Answer from the drawing. Dimensions are ordinates in mm from the lowest x, y and z of the part. Give positions to 0.01 mm unless a question says otherwise; leave off trailing zeros. Order: outer loops, then holes, each group sorted by start corner. A loop starts at its lowest first (then second) coordinate and runs counter-clockwise, first axis right, second up. Notation, with made-up numbers: M 2,40.5 L 60,40.5 A15 ccw 60,53.5 Z; hole C 82,-7.5 d5. An arc over 180 degrees is marked long. One line per item, written item: value.
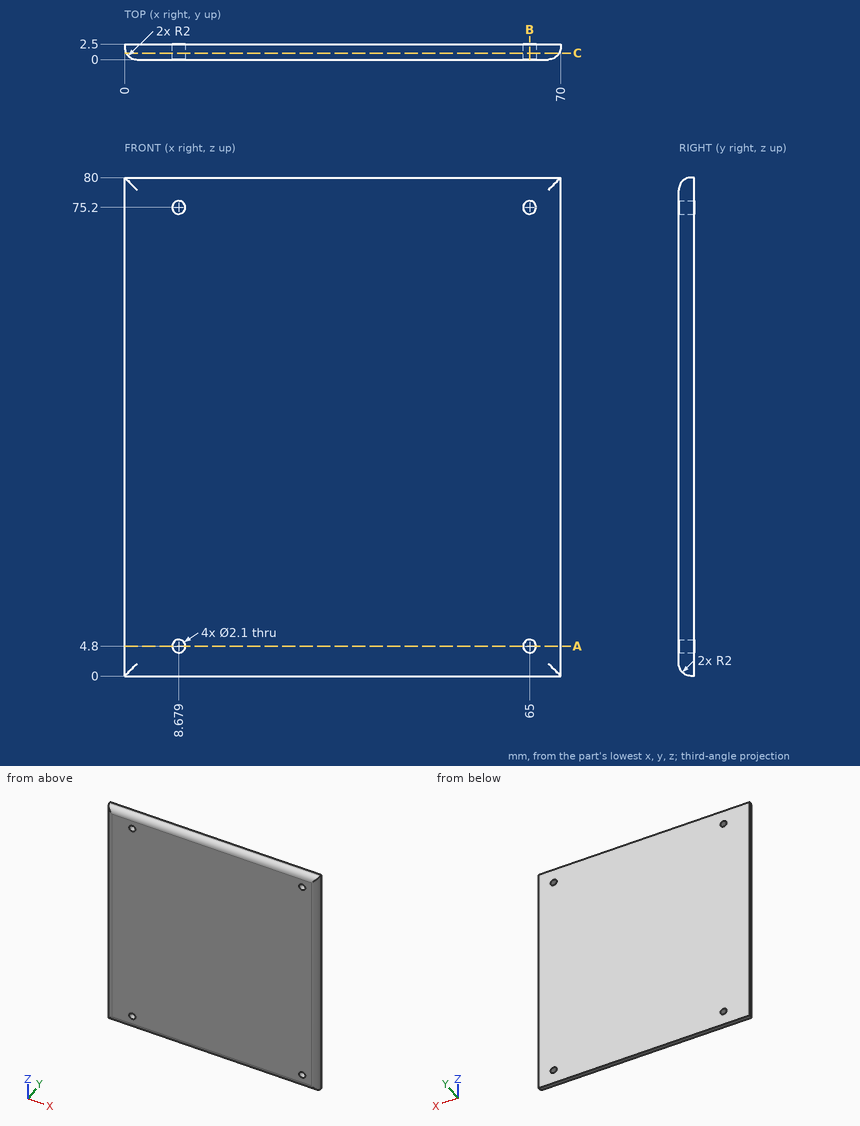
(1) Section B-B, the plane x = 65 is taken. Give the vertices of the cut face in (y, z), then the cut area to 3 significant figures.
Findings:
outline: M 0,2 A2 ccw 2,0 L 2.5,0 L 2.5,3.75 L 0,3.75 Z; M 0,5.85 L 2.5,5.85 L 2.5,74.15 L 0,74.15 Z; M 0,76.25 L 2.5,76.25 L 2.5,80 L 2,80 A2 ccw 0,78 Z
area: 188 mm^2
(2) Given P1, Ø3.5, axis at x = 65, z = 4.8, coming from the -Y side; P2, Ø1.5, axis at x = 18.5, y = 1, coming from the -Z side; P3, Ø1.5, axis at y = 0.5, z = 33, coming from the +X side, each flat-ended and moving along its own axis, determine where each tip first touches the part or whether it passes through.
Findings:
P1: stops at y = 0
P2: stops at z = 0.02
P3: stops at x = 69.85
(3) Section A-A, the plane z = 4.8 is taken. Give the vertices of the cut face in (x, y), then the cut area to 3 significant figures.
Findings:
outline: M 0,2 A2 ccw 2,0 L 7.63,0 L 7.63,2.5 L 0,2.5 Z; M 9.73,0 L 63.95,0 L 63.95,2.5 L 9.73,2.5 Z; M 66.05,0 L 68,0 A2 ccw 70,2 L 70,2.5 L 66.05,2.5 Z
area: 163 mm^2
(4) Find the intervals of material crossed by probe 1 along Z at (x, y) = (65, 1.8); probe 2 along X at (y, z) = (1.55, 75.2); probe 3 along Z at (x, y) = (65, 0.6), in increasing order. Write a range as from..to.
Findings:
probe 1: z = 0.01..3.75, 5.85..74.15, 76.25..79.99
probe 2: x = 0.05..7.63, 9.73..63.95, 66.05..69.95
probe 3: z = 0.57..3.75, 5.85..74.15, 76.25..79.43
(5) Section C-C, the plane y = 1.05 is taken. Give the vertices of the cut face in (x, z), then the cut area to 3 significant figures.
Findings:
outline: M 0.24,0.24 L 69.76,0.24 L 69.76,79.76 L 0.24,79.76 Z; hole C 8.68,4.8 d2.1; hole C 8.68,75.2 d2.1; hole C 65,4.8 d2.1; hole C 65,75.2 d2.1
area: 5,510 mm^2
